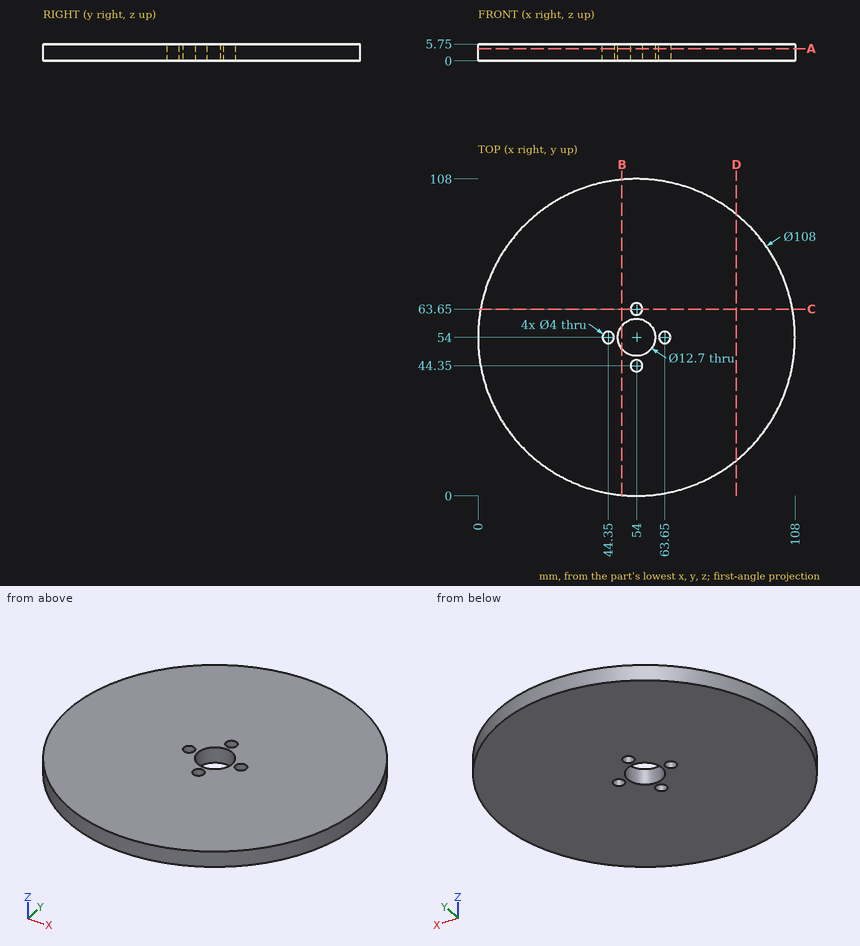
Source: three-view drawing plus pictorial views. Frame: mm from the lowest corner of the part. Coordinates: 2 decimals unless noted, no trailing zeros. Loops run counter-clockwise (first coordinate to the right, second up) from the corner with the lowest first, then second, coordinate; pieces in that order, holes last. Notation, with made-up numbers: (-13.75, 26) - (25.25, 26) arc R16 cw to (25.25, 44) - close; hole circle Ø6 at (-37.5, 16). An arc over 180 degrees is marked (long way). One line per item, written item: value. Start each with the question number.
1. Section B-B (x = 49). Return the cut outline in (y, z), and give its area (3 significant figures).
2. Ray query, L1, parallel to Y at x = 54, z = 3.7; L2, parallel to Y at x = 46, z = 2.1; L3, parallel to Y at x = 44.35, z = 2.8. Return the intervals inside material, ascending.
3. Section A-A (z = 4.2). Return the cut outline in (x, y).
4. Section C-C (y = 63.65). Return the cut outline in (x, z).
5. Section D-D (x = 88). Return the cut outline in (y, z), and give its area (3 significant figures).
6. Contact query for flat-ended pins moving along their axis: P1, Ø1.5, axis at x = 32.5, z = 5, coming from the -Y side; P2, Ø1.5, axis at y = 30, z = 2.5, coming from the -X side; P3, Ø3, axis at x = 34.5, z = 4, coming from the +Y side. Output: stop coordinate, or through.
Verdict:
1. outline: (0.23, 0) - (50.09, 0) - (50.09, 5.75) - (0.23, 5.75) - close; (57.91, 0) - (107.77, 0) - (107.77, 5.75) - (57.91, 5.75) - close
1. area: 573 mm2
2. L1: y = 0 to 42.35, 46.35 to 47.65, 60.35 to 61.65, 65.65 to 108
2. L2: y = 0.6 to 52.87, 55.13 to 107.4
2. L3: y = 0.87 to 52, 56 to 107.13
3. outline: circle Ø108 at (54, 54); hole circle Ø4 at (44.35, 54); hole circle Ø12.7 at (54, 54); hole circle Ø4 at (54, 44.35); hole circle Ø4 at (54, 63.65); hole circle Ø4 at (63.65, 54)
4. outline: (0.87, 0) - (52, 0) - (52, 5.75) - (0.87, 5.75) - close; (56, 0) - (107.13, 0) - (107.13, 5.75) - (56, 5.75) - close
5. outline: (12.05, 0) - (95.95, 0) - (95.95, 5.75) - (12.05, 5.75) - close
5. area: 482 mm2
6. P1: stops at y = 4.15
6. P2: stops at x = 5.26
6. P3: stops at y = 104.91
